```python
from build123d import *

# Parameters (mm, degrees)
SKETCH1_W                    = 127
SKETCH1_H                    = 38.1
BOSS_EXTRUDE1_DEPTH          = 19.05
BOSS_EXTRUDE2_DEPTH          = 6.35
FILLET1_R                    = 12.7
SKETCH3_R                    = 19.05
BOSS_EXTRUDE3_DEPTH          = 6.35
BOSS_EXTRUDE4_DEPTH          = 12.7
BOSS_EXTRUDE6_DEPTH          = 12.7
F_3_8_1_25_DIAMETER_HOLE1_D  = 31.75
F_1_4_20_TAPPED_HOLE1_D      = 5.1054
SKETCH11_R                   = 3.175
CUT_EXTRUDE1_DEPTH           = 19.05
F_1_4_0_356_DIAMETER_HOLE1_D = 9.0424
F_1_4_0_75_DIAMETER_HOLE1_D  = 19.05
SKETCH16_R                   = 2.413
BOSS_EXTRUDE7_DEPTH          = 6.35
CHAMFER1_SIZE                = 0.762


with BuildPart() as part:
    # Sketch1 → Boss-Extrude1 (new body)
    with BuildSketch(Plane(origin=(0, 0, 0), x_dir=(1, 0, 0), z_dir=(0, 1, 0))):
        with Locations((63.5, 19.05)):
            Rectangle(SKETCH1_W, SKETCH1_H)
    extrude(amount=-BOSS_EXTRUDE1_DEPTH)

    # Sketch2 → Boss-Extrude2 (add)
    with BuildSketch(Plane(origin=(0, 0, 0), x_dir=(1, 0, 0), z_dir=(0, 1, 0))):
        with BuildLine():
            Line((28.361415, 0), (98.638585, 0))
            Line((98.638585, 0), (81.099905, -42.342119))
            ThreePointArc((81.099905, -42.342119), (63.5, -54.102), (45.900095, -42.342119))
            Line((45.900095, -42.342119), (28.361415, 0))
        make_face()
    extrude(amount=-BOSS_EXTRUDE2_DEPTH)

    # Fillet1
    fillet1_edges = [part.edges().sort_by_distance(p)[0] for p in [
        (28.361415, -3.175, 0),
        (98.638585, -3.175, 0),
    ]]
    fillet(fillet1_edges, radius=FILLET1_R)

    # Sketch3 → Boss-Extrude3 (add, symmetric)
    with BuildSketch(Plane(origin=(0, -3.175, 0), x_dir=(1, 0, 0), z_dir=(0, 1, 0))):
        with Locations(Location((63.5, -35.052, 0), (0, 0, 270))):
            Circle(SKETCH3_R)
    extrude(amount=BOSS_EXTRUDE3_DEPTH, both=True)

    # Sketch4 → Boss-Extrude4 (add)
    with BuildSketch(Plane.XY.offset(-38.1)):
        with BuildLine():
            Line((0, 0), (0, 50.8))
            ThreePointArc((0, 50.8), (5.579616, 64.270384), (19.05, 69.85))
            Line((19.05, 69.85), (57.15, 69.85))
            ThreePointArc((57.15, 69.85), (65.01503, 68.150614), (71.476835, 63.355648))
            Line((71.476835, 63.355648), (127, 0))
            Line((127, 0), (0, 0))
        make_face()
    extrude(amount=BOSS_EXTRUDE4_DEPTH)

    # Sketch7 → Boss-Extrude6 (add, symmetric)
    with BuildSketch(Plane.XY.offset(-31.75)):
        with BuildLine():
            Line((19.05, 69.85), (57.15, 69.85))
            ThreePointArc((57.15, 69.85), (76.2, 50.8), (57.15, 31.75))
            Line((57.15, 31.75), (19.05, 31.75))
            ThreePointArc((19.05, 31.75), (0, 50.8), (19.05, 69.85))
        make_face()
    extrude(amount=BOSS_EXTRUDE6_DEPTH, both=True)

    # 3/8 (1.25) Diameter Hole1 (through all)
    with Locations(Plane(origin=(19.05, 50.8, -19.05), x_dir=(1, 0, 0), z_dir=(0, 0, 1))):
        with Locations((0, 0), (38.1, 0)):
            Hole(F_3_8_1_25_DIAMETER_HOLE1_D / 2)

    # 1/4-20 Tapped Hole1 (through all)
    with Locations(Plane(origin=(12.7, -9.525, 0), x_dir=(1, 0, 0), z_dir=(0, 0, 1))):
        with Locations((0, 0), (101.6, 0)):
            Hole(F_1_4_20_TAPPED_HOLE1_D / 2)

    # Sketch11 → Cut-Extrude1 (cut)
    with BuildSketch(Plane.XY.offset(54.61)):
        with Locations((63.5, -3.175)):
            Circle(SKETCH11_R)
    extrude(amount=-CUT_EXTRUDE1_DEPTH, mode=Mode.SUBTRACT)

    # 1/4 (0.356) Diameter Hole1 (through all)
    with Locations(Plane(origin=(127, -9.398, -15.748), x_dir=(0, 0, 1), z_dir=(1, 0, 0))):
        with Locations((0, 0)):
            Hole(F_1_4_0_356_DIAMETER_HOLE1_D / 2)

    # 1/4 (0.75) Diameter Hole1 (through all)
    with Locations(Plane(origin=(63.5, 3.175, 35.052), x_dir=(0, 0, 1), z_dir=(0, 1, 0))):
        with Locations((0, 0)):
            Hole(F_1_4_0_75_DIAMETER_HOLE1_D / 2)

    # Sketch16 → Boss-Extrude7 (add)
    with BuildSketch(Plane(origin=(0, 3.175, 0), x_dir=(1, 0, 0), z_dir=(0, 1, 0))):
        with Locations(Location((63.5, -20.7645, 0), (0, 0, 270))):
            Circle(SKETCH16_R)
        with Locations(Location((74.670417, -26.143889, 0), (0, 0, 270))):
            Circle(SKETCH16_R)
        with Locations(Location((77.429283, -38.231268, 0), (0, 0, 270))):
            Circle(SKETCH16_R)
        with Locations(Location((69.699114, -47.924593, 0), (0, 0, 270))):
            Circle(SKETCH16_R)
        with Locations(Location((57.300886, -47.924593, 0), (0, 0, 270))):
            Circle(SKETCH16_R)
        with Locations(Location((49.570717, -38.231268, 0), (0, 0, 270))):
            Circle(SKETCH16_R)
        with Locations(Location((52.329583, -26.143889, 0), (0, 0, 270))):
            Circle(SKETCH16_R)
    extrude(amount=BOSS_EXTRUDE7_DEPTH)

    # Chamfer1
    chamfer1_edges = [part.edges().sort_by_distance(p)[0] for p in [
        (63.5, 9.525, 18.3515),
        (74.670417, 9.525, 23.730889),
        (77.429283, 9.525, 35.818268),
        (69.699114, 9.525, 45.511593),
        (57.300886, 9.525, 45.511593),
        (49.570717, 9.525, 35.818268),
        (52.329583, 9.525, 23.730889),
    ]]
    chamfer(chamfer1_edges, length=CHAMFER1_SIZE)


solid = part.part
```
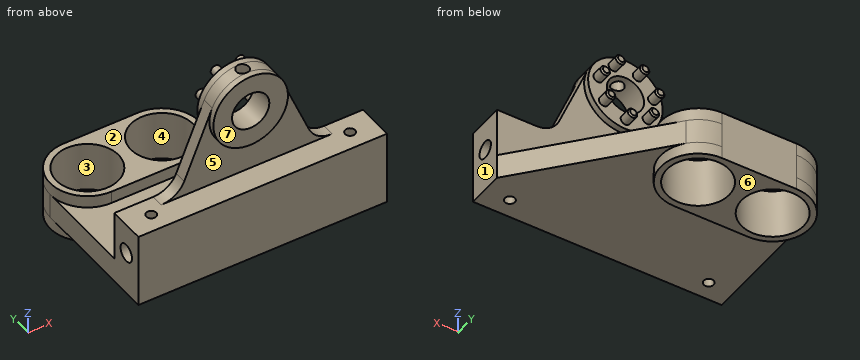
Part model, mm, in its own coordinate system. Face numbers are marked on the shaded views. A direction names the side the tool comes from. Round coordinates to 2 decimals unless told otherwise and drop trailing zeros. Order: outer loops, then holes, each group sorted by start corner. A loop starts at its lowest first (then second) coordinate and runs counter-clockwise, first axis right, second up. Notation, with made-up numbers: M -10,4.5 L 38,4.5 A10 cw 38,8.5 Z; hole C 56,74 d4. An arc over 180 degrees is marked long. Put each result on its own line as item: value. Start each with the question number.
1. Slice it at C-C on x = 12.7. List the corners of the cut face in (y, z).
2. Two-plate mould, pull along X, no slides. Class the marked faces 1, 2, 3 and 4: +X half, -X half, draft (parallel to the pull), parting line (faces both ways), or undercut.
3. Slice it at B-B on y = 47. List the corners of the cut face in (x, z).
4. Slice it at D-D on z = 1.5. List the corners of the cut face in (x, y), then the cut area to 3 significant figures.
5. Drill centre lines: probe 1 along Y at (x, z) = (114, -25); probe 2 along X at (y, z) = (-9, -5); probe 3 along X at (y, z) = (-11, -38). Where is each one in solid material? Low to high. Write a range as [from, to].
6. Tool access for the marked faces 5, 6 and 7: list every direction of +Z, -Z, +X, -X, +Y, -Y with a clear straight run to the whole face (end or side of a thin tool).
7. Drop flat-ended pins along their axis: pin 1 (3.5 mm diameter, centred on x = 50, z = 39, fed in from +Y) (3 decimals); pin 2 (3 mm diameter, centred on x = 74.5, y = 45, fed in from +Z); pin 3 (6 mm diameter, centred on x = 114.3, y = -9.525, fed in from +Z); pin 4 (19 mm diameter, centred on x = 19.05, y = 50.8, fed in from +Z). Give the stop position or say it passes through.
8. Slice it at A-A on x = 109.5. List the corners of the cut face in (y, z).
Findings:
1. outline: M -19.05,-38.1 L -12.08,-38.1 L -12.08,-19.39 A4.52 cw -12.08,-12.11 L -12.08,0 L -19.05,0 Z; M -6.97,-38.1 L 32.84,-38.1 L 32.84,-44.45 L 36.25,-44.45 L 36.25,-19.05 L 32.84,-19.05 L 32.84,-25.4 L 0,-25.4 L 0,0 L -6.97,0 L -6.97,-11.93 A4.52 cw -6.97,-19.56 Z; M 65.35,-44.45 L 68.76,-44.45 L 68.76,-19.05 L 65.35,-19.05 Z
2. face 1: +X half
2. face 2: draft
2. face 3: undercut
2. face 4: undercut
3. outline: M 0,-38.1 L 0.38,-38.1 L 0.38,-44.45 L 3.64,-44.45 L 3.64,-19.05 L 0.38,-19.05 L 0.38,-25.4 L 0,-25.4 Z; M 34.46,-44.45 L 41.74,-44.45 L 41.74,-19.05 L 34.46,-19.05 Z; M 72.56,-44.45 L 75.82,-44.45 L 75.82,-38.1 L 85.81,-38.1 L 85.81,-25.4 L 75.82,-25.4 L 75.82,-19.05 L 72.56,-19.05 Z
4. outline: M 25.86,-6.35 L 101.14,-6.35 L 101.14,0 L 25.86,0 Z
4. area: 478 mm2
5. probe 1: [-19.05, -12.06], [-6.99, 0]
5. probe 2: [0, 10.2], [15.2, 111.8], [116.8, 127]
5. probe 3: [0, 10.62], [14.78, 112.22], [116.38, 127]
6. face 5: -Y
6. face 6: -Z, +X, -X, +Y, -Y
6. face 7: +Z, +X, -X, -Y
7. pin 1: y = 9.525
7. pin 2: z = -19.05
7. pin 3: z = 0
7. pin 4: through
8. outline: M -19.05,-38.1 L 19.97,-38.1 L 19.97,-25.4 L 0,-25.4 L 0,0 L -19.05,0 Z; hole C -9.4,-15.75 d9.04
